```python
from build123d import *

# Parameters (mm, degrees)
F0_R     = 6.3836352682
F1_DEPTH = 171.45
F4_R     = 5.1492450533
F5_DEPTH = 171.45
F6_DEPTH = 12.7
F6_TAPER = 14
F8_DEPTH = 25.654


# Not quite as in the source:
# - the program builds the solid bodies; features that only make, move or delete a surface that nothing else refers to are left out


with BuildPart() as f1:
    # F0 (on Front) → F1 (new body)
    with BuildSketch(Plane.XZ):
        with Locations((-119.9116557837, -45.1905839145)):
            Circle(F0_R)
    extrude(amount=F1_DEPTH)

    # F4 (on Front) → F5 (cut)
    with BuildSketch(Plane.XZ):
        with Locations((-119.9116557837, -45.1905839145)):
            Circle(F4_R)
    extrude(amount=F5_DEPTH, mode=Mode.SUBTRACT)

    # F0 (on Front) → F6 (join)
    with BuildSketch(Plane.XZ):
        with Locations((-119.9116557837, -45.1905839145)):
            Circle(F0_R)
    extrude(amount=-F6_DEPTH, taper=F6_TAPER)

    # F8 (cut): a face of the model
    f8_faces = [f1.faces().sort_by_distance(p)[0] for p in [
        (-119.9116557837, 12.7, -45.1905839145),
    ]]
    extrude(f8_faces, amount=-F8_DEPTH, mode=Mode.SUBTRACT)


solid = f1.part
```
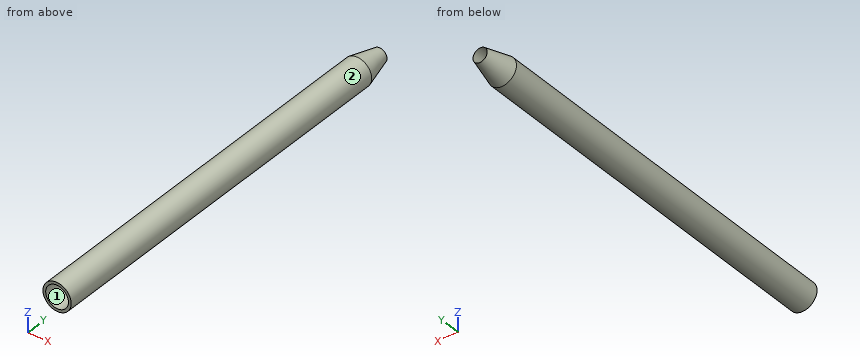
Verification items for the finished model (mm, model axes). Face numbers are marked on the shaded views. Coordinates: 2 decimals unless noted, no trailing zeros. Loops run counter-clockwise (first coordinate to the right, second up) from the corner with the lowest first, then second, coordinate; pieces in that order, holes last. Notation, with made-up numbers: (62, -1.75) - (79, -1.75) arc R12 cw to (79, 19.25) - close; hole circle Ø4 at (-36.5, -7.5). An arc over 180 degrees is marked (long way). Answer as a JSON object with one key per item and string values.
(1) Cross-section at A-A, the plane y = -45. Record the boundary of the cut face in (x, z), then the cut area to 3 significant figures.
Response:
{"outline": "circle Ø12.77 at (-119.91, -45.19); hole circle Ø10.3 at (-119.91, -45.19)", "area": "44.7 mm²"}
(2) Scan lines: line 1 along Z through (x, y) = (-120.25, -104.5); line 2 along Z through (x, y) = (-120.5, -51.5); line 3 along X through (y, z) = (-66.5, -42.5). Record each from-to range of solid material in increasing order.
Response:
{"line 1": "z = -51.57 to -50.33, -40.05 to -38.82", "line 2": "z = -51.55 to -50.31, -40.08 to -38.83", "line 3": "x = -125.7 to -124.3, -115.52 to -114.12"}
(3) Go/stop test with flat-tipped pins: pin 1 Ø6 at (y, z) = (-63.5, -48.5) entering from -X; pin 2 Ø7.5 at (x, z) = (-119.91, -45.19) entering from -Y; pin 3 Ø2 at (x, y) = (-117, -57) entering from +Z. Record where each tip stops, or that it passes through.
Response:
{"pin 1": "stops at x = -126.29", "pin 2": "stops at y = 0", "pin 3": "stops at z = -39.1"}
(4) Mould release check, pull along X, two halves, no side actions. Record for the marked faces 1 and 2: pulls with the +X half, pulls with the -X half, needs draft (parallel to the pull), parting line crosses it, or undercut.
Response:
{"face 1": "undercut", "face 2": "parting line crosses it"}
